The model under review builds one solid part; all positions refer to its coordinate system, in mm. A direction names the side the tool comes from. Give positions to 0.01 mm unless a question says otherwise; leave off trailing zeros. Loops run counter-clockwise (first coordinate to the right, second up) from the corner with the lowest first, then second, coordinate; pieces in that order, holes last. Notation, with made-up numbers: (74, 57.5) -> (82, 57.5) arc R14 ccw to (82, 72.5) -> close; hole circle Ø10 at (11.5, 86.5). An arc over 180 degrees is marked (long way). Write each question's results on one line, items separated by ' | '. Start each with the question number.
Q1. We need section C-C (z = 3.75). Write out the cut boundary in (x, y) (3 decimals), plus the area to 3 significant figures.
Q2. Wall thickness on L1, parallel to Z at x = 0.5, y = -2.15 (3 decimals); L2, parallel to X at y = -1, z = 11.25; L3, parallel to X at y = 1.3, z = 10: over which ranges is each line inside the solid? List them lowest first. Write a range as [from, to].
Q3. We need section B-B (x = 0). Write out the cut boundary in (y, z) (3 decimals), plus the area to 3 significant figures.
Q4. We need section A-A (y = 0). Write out the cut boundary in (x, z) (3 decimals), plus the area to 3 significant figures.
Q5. Machinability: for faces 1 (the face through (-2.85, 0.04, 1.35)), 2 (the face through (-3.31, 0.019, -0.355)), 3 (the face through (-1.5, 0, 9)), 4 (the face through (1.5, 0, 9)), 5 (the face through (2.88, 0.04, 1.35)), which of the approach directions +Z, -Z, +X, -X, +Y, -Y give a long, thin tool a straight path to every point of the face, cutting with its end or side? Answer none if there is none.
Q6. Insertion check: pin 1 Ø2.5 at (y, z) = (0, 10) entering from +X; pin 2 Ø1.1 at (y, z) = (-0.5, 8.5) entering from -X; pin 3 Ø0.5 at (y, z) = (-2.5, 0) entering from -X (3 decimals). Each pin has a flat end and moves straight along its axis. Give the tip position at first contact, or say it passes through.
Q7. We need section D-D (x = -2.5). Write out the cut boundary in (y, z).
from build123d import *

# Parameters (mm, degrees)
SKETCH001_R          = 1.875
PAD_DEPTH            = 6.5
PAD002_DEPTH         = 5
SKETCH002_R          = 1.35
PAD001_DEPTH         = 3.925
POCKET_DEPTH         = 1.876
POCKET_DEPTH_BACK    = 1.876
SKETCH005_W          = 1.35
SKETCH005_H          = 1.7
PAD003_DEPTH         = 2.8
POCKET001_DEPTH      = 3.926
POCKET001_DEPTH_BACK = 3.926


with BuildPart() as part:
    # Sketch001 → Pad (new body)
    with BuildSketch(Plane.XY):
        Circle(SKETCH001_R)
    extrude(amount=PAD_DEPTH)

    # Sketch003 → Pad002 (join)
    with BuildSketch(Plane.XY.offset(6.5)):
        with BuildLine():
            ThreePointArc((1.5, 1.125), (1.392997, 1.255063), (1.274755, 1.375))
            Line((0.5, 1.375), (1.274755, 1.375))
            Line((0.5, 1.807104), (0.5, 1.375))
            ThreePointArc((0.5, 1.807104), (0, 1.875), (-0.5, 1.807104))
            Line((-0.5, 1.807104), (-0.5, 1.375))
            Line((-1.274755, 1.375), (-0.5, 1.375))
            ThreePointArc((-1.274755, 1.375), (-1.392997, 1.255063), (-1.5, 1.125))
            Line((-1.5, 1.125), (-1.5, -1.125))
            ThreePointArc((-1.5, -1.125), (0, -1.875), (1.5, -1.125))
            Line((1.5, 1.125), (1.5, -1.125))
        make_face()
    extrude(amount=PAD002_DEPTH)

    # Sketch002 → Pad001 (join, symmetric)
    with BuildSketch(Plane.YZ):
        Circle(SKETCH002_R)
    extrude(amount=PAD001_DEPTH, both=True)

    # Sketch004 → Pocket (cut, two sides)
    with BuildSketch(Plane.XZ) as pocket_sk:
        Polygon((-3.925, 0), (-3.925, -3), (3.925, -3), (3.925, 0), (2.712564, -0.7), (-2.712564, -0.7), align=None)
    extrude(amount=-POCKET_DEPTH, mode=Mode.SUBTRACT)
    extrude(pocket_sk.sketch, amount=POCKET_DEPTH_BACK, mode=Mode.SUBTRACT)

    # Sketch → Revolution (revolve)
    with BuildSketch(Plane.XY):
        with BuildLine():
            ThreePointArc((0, -2.25), (2.25, 0), (0, 2.25))
            Line((0, 2.25), (0, -2.25))
        make_face()
    revolve(axis=Axis((0, 0, 0), (0, 1, 0)))

    # Sketch005 → Pad003 (join)
    with BuildSketch(Plane.XZ):
        with Locations((0, 0.175)):
            Rectangle(SKETCH005_W, SKETCH005_H)
    extrude(amount=PAD003_DEPTH)

    # Sketch006 → Pocket001 (cut, two sides)
    with BuildSketch(Plane.YZ) as pocket001_sk:
        with BuildLine():
            Line((-2.8, 0.15), (-3.062142, 0.15))
            Line((-3.062142, 0.15), (-3.062142, 1.35))
            Line((-3.062142, 1.35), (-2.462142, 1.35))
            ThreePointArc((-2.462142, 1.35), (-2.713925, 0.773327), (-2.8, 0.15))
        make_face()
    extrude(amount=-POCKET001_DEPTH, mode=Mode.SUBTRACT)
    extrude(pocket001_sk.sketch, amount=POCKET001_DEPTH_BACK, mode=Mode.SUBTRACT)


solid = part.part
Output:
1) outline: circle Ø3.75 at (0, 0) | area: 11.0 mm2
2) L1: [-0.675, 1.025] | L2: [-1.5, 1.5] | L3: [-1.35, 1.35]
3) outline: (-2.8, -0.675) -> (-2.146, -0.675) arc R2.25 ccw (long way) to (1.875, 1.244) -> (1.875, 11.5) -> (-1.875, 11.5) -> (-1.875, 1.244) arc R2.25 ccw to (-2.003, 1.025) -> (-2.627, 1.025) arc R2.3 ccw to (-2.8, 0.15) -> close | area: 52.7 mm2
4) outline: (-3.925, 0) -> (-2.713, -0.7) -> (-2.138, -0.7) arc R2.25 ccw to (2.138, -0.7) -> (2.713, -0.7) -> (3.925, 0) -> (3.925, 1.35) -> (1.875, 1.35) -> (1.875, 6.5) -> (1.5, 6.5) -> (1.5, 11.5) -> (-1.5, 11.5) -> (-1.5, 6.5) -> (-1.875, 6.5) -> (-1.875, 1.35) -> (-3.925, 1.35) -> close | area: 54.4 mm2
5) face 1: -X | face 2: -Z, -X, +Y, -Y | face 3: +Z, -X, +Y, -Y | face 4: +Z, +X, +Y, -Y | face 5: +X
6) pin 1: x = 1.5 | pin 2: x = -1.5 | pin 3: x = -0.675
7) outline: (-1.15, -0.7) -> (1.15, -0.7) arc R1.35 ccw (long way) to start
